Part model, mm, in its own coordinate system. Face numbers are marked on the shaded views. A direction names the side the tool comes from. Round coordinates to 2 decimals unless told otherwise and drop trailing zeros. Write each loop counter-clockwise with the first axis right and the second up, starting at its lowest first coordinate (ties: lowest second). Pieces come first, ordered by that corner, then holes. Notation, with made-up numbers: (27, 19.25) -> (84, 19.25) arc R19 ccw to (84, 39.25) -> close; hole circle Ø11 at (-19.75, 26). An arc over 180 degrees is marked (long way). Use CSV: the item, a comma, the result in double quotes. Start each with the question number.
(1) Saw through at A-A (z = 1.5). Give the cut face in (x, y), plus the area to 3 significant figures.
(2) Which spindle directions (+Z, -Z, +X, -X, +Y, -Y) get a long thin tool onto all of the face, cutting with end or side? Do the marked faces 4, 5, 6 and 7. Say none if no direction does.
(3) Probe line 1 (Y direction, x = 3.75, z = -2.25); line 2 (Y direction, x = -4.5, z = 0.25); line 3 (X direction, y = 17.5, z = 0.25). List the from-to ranges inside material, lowest first. Write a range as [from, to].
(4) Two-plate mould, pull along Y, no slides. Class the marked faces 1, 2 and 3: released by +Y, released by -Y, zero draft, split by the parting line, or undercut.
(5) Drop flat-ended pins along their axis: pin 1 (5.5 mm diameter, centred on x = -3.5, z = 3, fed in from -Y); pin 2 (1.5 mm diameter, centred on x = 3, z = -3.5, fed in from -Y); pin 3 (1 mm diameter, centred on x = 4.5, z = -2.5, fed in from +Y). Give the stop position or say it passes through.
(6) Saw through at B-B (x = 3.81). Give the cut face in (y, z).
(7) Saw through at C-C (y = 20.32). Give the cut face in (x, z).
(8) Saw through at D-D (z = -3.75). Give the cut face in (x, y), plus the area to 3 significant figures.
```python
from build123d import *

# Parameters (mm, degrees)
BOSS_EXTRUDE1_DEPTH = 5.08
SKETCH2_R           = 1.27
BOSS_EXTRUDE2_DEPTH = 5.08


with BuildPart() as part:
    # Sketch1 → Boss-Extrude1 (new body)
    with BuildSketch(Plane.XY):
        Polygon((0, 0), (0, 22.86), (-7.62, 22.86), (-7.62, 30.48), (0, 30.48), (0, 38.1), (7.62, 38.1), (7.62, 30.48), (15.24, 30.48), (15.24, 22.86), (7.62, 22.86), (7.62, 0), align=None)
    extrude(amount=BOSS_EXTRUDE1_DEPTH)

    # Sketch2 → Boss-Extrude2 (add)
    with BuildSketch(Plane(origin=(0, 0, 0), x_dir=(-1, 0, 0), z_dir=(0, 0, -1))):
        with Locations((-3.81, 20.32)):
            Circle(SKETCH2_R)
        with Locations((-3.81, 12.7)):
            Circle(SKETCH2_R)
    extrude(amount=BOSS_EXTRUDE2_DEPTH)


solid = part.part
```
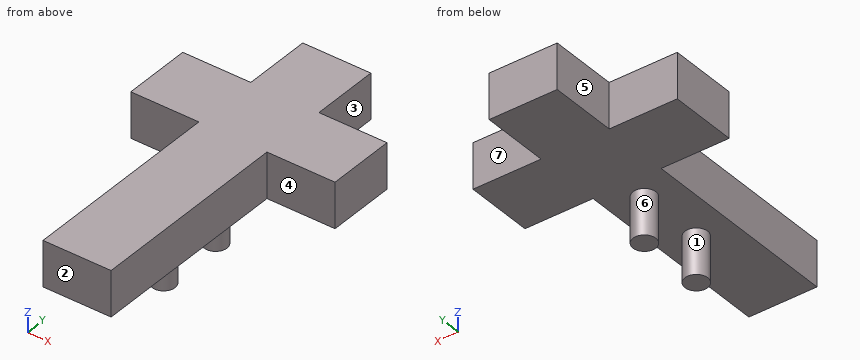
Answers:
1,outline,"(-7.62, 22.86) -> (0, 22.86) -> (0, 0) -> (7.62, 0) -> (7.62, 22.86) -> (15.24, 22.86) -> (15.24, 30.48) -> (7.62, 30.48) -> (7.62, 38.1) -> (0, 38.1) -> (0, 30.48) -> (-7.62, 30.48) -> close"
1,area,"406 mm²"
2,face 4,"+Z, -Z, +X, -Y"
2,face 5,"+Z, -Z, -X, +Y"
2,face 6,"-Z"
2,face 7,"+Z, -Z, +X, +Y"
3,line 1,"y = [11.43, 13.97], [19.05, 21.59]"
3,line 2,"y = [22.86, 30.48]"
3,line 3,"x = [0, 7.62]"
4,face 1,"undercut"
4,face 2,"released by -Y"
4,face 3,"zero draft"
5,pin 1,"stops at y = 22.86"
5,pin 2,"stops at y = 11.43"
5,pin 3,"stops at y = 21.58"
6,outline,"(0, 0) -> (11.43, 0) -> (11.43, -5.08) -> (13.97, -5.08) -> (13.97, 0) -> (19.05, 0) -> (19.05, -5.08) -> (21.59, -5.08) -> (21.59, 0) -> (38.1, 0) -> (38.1, 5.08) -> (0, 5.08) -> close"
7,outline,"(0, 0) -> (2.54, 0) -> (2.54, -5.08) -> (5.08, -5.08) -> (5.08, 0) -> (7.62, 0) -> (7.62, 5.08) -> (0, 5.08) -> close"
8,outline,"circle Ø2.54 at (3.81, 12.7); circle Ø2.54 at (3.81, 20.32)"
8,area,"10.1 mm²"
